Check sheet for the modelled part. Datum: model origin and axes. Units: mm. A direction names the side the tool comes from. Give positions to 0.01 mm unless a question says otherwise; leave off trailing zeros. Order: outer loops, then holes, each group sorted by start corner. A loop starts at its lowest first (then second) coordinate and runs counter-clockwise, first axis right, second up.
from build123d import *

# Parameters (mm, degrees)
F1_DEPTH     = 16.25
F2_DEPTH     = 25
F3_START     = 24
F3_DEPTH     = 1
F4_START     = 17
F4_DEPTH     = 8
F5_T1_DEPTH  = 88.2485217467
F5_T3_DEPTH  = 96.2485217467
F5_T5_DEPTH  = 88.9985217467
F5_T10_DEPTH = 96.5839074706
F5_T15_DEPTH = 88.4985217467
F5_T20_DEPTH = 86.4985217467
F5_T23_ANGLE = 359.64
F5_T25_ANGLE = 359.64


# Not quite as in the source:
# - a fillet or chamfer that OpenCascade refuses, or shapes differently, is made with other operations: its cross-section is extruded or revolved along the edge and cut away or added


with BuildPart() as f1:
    # F0 (on Top) → F1 (new body)
    with BuildSketch(Plane.XY):
        with BuildLine():
            Line((-8.75, -5.75), (-7, -5.75))
            Line((-7, -5.75), (-7, 6.3353857239))
            Line((-7, 6.3353857239), (-9.0223743914, 8.3577601154))
            Line((-9.0223743914, 8.3577601154), (-9.0223743914, 14.1793463062))
            Line((-9.0223743914, 14.1793463062), (-5.6981157623, 15.6555524338))
            Line((-5.6981157623, 15.6555524338), (-1.1670593175, 5.4520969645))
            Line((-1.1670593175, 5.4520969645), (-5, 3.75))
            Line((-5, 3.75), (-5, 1.75))
            ThreePointArc((-5, 1.75), (-3.7625631329, 1.2374368671), (-3.25, 0))
            ThreePointArc((-3.25, 0), (-3.7625631329, -1.2374368671), (-5, -1.75))
            Line((-5, -1.75), (-5, -5.75))
            Line((-5, -5.75), (-2, -5.75))
            Line((-2, -5.75), (-2, -6.25))
            Line((-2, -6.25), (-1, -6.25))
            Line((-1, -6.25), (-1, 10.0037865203))
            Line((-1, 10.0037865203), (-6.1024322628, 21.4939193431))
            Line((-6.1024322628, 21.4939193431), (-12.5, 18.652946438))
            Line((-12.5, 18.652946438), (-12.5, 0.25))
            Line((-12.5, 0.25), (-8.75, 0.25))
            Line((-8.75, 0.25), (-8.75, -5.75))
        make_face()
    extrude(amount=F1_DEPTH)

    # F0 (on Top) → F2 (join)
    with BuildSketch(Plane.XY):
        Polygon((1, 5.5), (-1, 10.0037865203), (-1, -6.25), (1, -6.25), align=None)
    extrude(amount=F2_DEPTH)



with BuildPart() as f2:
    # F0 (on Top) → F2, piece 2 (new body)
    with BuildSketch(Plane.XY):
        with BuildLine():
            Line((6, 5.5), (3, 5.5))
            Line((3, 5.5), (3, 1.75))
            ThreePointArc((3, 1.75), (4.75, 0), (3, -1.75))
            Line((3, -1.75), (3, -6.25))
            Line((3, -6.25), (6, -6.25))
            Line((6, -6.25), (6, 5.5))
        make_face()
    extrude(amount=F2_DEPTH)


with BuildPart() as f1_1:
    add(f1.part)

    add(f2.part)  # F3 merges F2
    # F0 (on Top) → F3 (join)
    with BuildSketch(Plane.XY.offset(F3_START)):
        Polygon((3, 5.5), (1, 5.5), (1, -6.25), (3, -6.25), (3, -1.75), (3, 1.75), align=None)
    extrude(amount=F3_DEPTH)

    # F0 (on Top) → F4 (join)
    with BuildSketch(Plane.XY.offset(F4_START)):
        with BuildLine():
            ThreePointArc((3, -1.75), (4.75, 0), (3, 1.75))
            Line((3, 1.75), (3, -1.75))
        make_face()
    extrude(amount=F4_DEPTH)

    # F5: chamfer of 16.25 x 0.5 on 8 edges, made by hand

    # F5_s2 → F5_t1 (cut)
    with BuildSketch(Plane.XZ.offset(-47.7492608733)):
        Polygon((3.5, 0), (3, 16.25), (3, 0), align=None)
    extrude(amount=F5_T1_DEPTH, mode=Mode.SUBTRACT)

    # F5_s4 → F5_t3 (cut)
    with BuildSketch(Plane.XZ.offset(-47.7492608733)):
        Polygon((0.5, 0), (1, 16.25), (1, 0), align=None)
    extrude(amount=F5_T3_DEPTH, mode=Mode.SUBTRACT)

    # F5_s6 → F5_t5 (cut)
    with BuildSketch(Plane.XZ.offset(-40.4992608733)):
        Polygon((3.5, 0), (3, 16.25), (3, 0), align=None)
    extrude(amount=F5_T5_DEPTH, mode=Mode.SUBTRACT)


with BuildPart() as f5_tool8:
    # F5_s9 → F5_t10 (new body)
    with BuildSketch(Plane.XZ.offset(47.9992608733)):
        Polygon((-7, 16.25), (-7.5, 0), (-7, 0), align=None)
    extrude(amount=-F5_T10_DEPTH)

    split(bisect_by=Plane(origin=(-0.332307138, -0.332307138, 0), x_dir=(0, 0, 1), z_dir=(-0.7071067812, -0.7071067812, 0)), keep=Keep.TOP)


with BuildPart() as f1_2:
    add(f1_1.part)

    # F5_t7: cut F5_tool8
    add(f5_tool8.part, mode=Mode.SUBTRACT)


with BuildPart() as f5_tool13:
    # F5_s14 → F5_t15 (new body)
    with BuildSketch(Plane.XZ.offset(-40.4992608733)):
        Polygon((-5, 16.25), (-4.5, 0), (-5, 0), align=None)
    extrude(amount=F5_T15_DEPTH)

    split(bisect_by=Plane(origin=(1.0474931823, 0.4651611161, 0), x_dir=(0, 0, 1), z_dir=(-0.9139382482, -0.4058532722, 0)), keep=Keep.TOP)


with BuildPart() as f1_3:
    add(f1_2.part)

    # F5_t12: cut F5_tool13
    add(f5_tool13.part, mode=Mode.SUBTRACT)


with BuildPart() as f5_tool18:
    # F5_s19 → F5_t20 (new body)
    with BuildSketch(Plane.XZ.offset(-45.9992608733)):
        Polygon((-5, 16.25), (-4.5, 0), (-5, 0), align=None)
    extrude(amount=F5_T20_DEPTH)

    split(bisect_by=Plane(origin=(1.0474931823, 0.4651611161, 0), x_dir=(0, 0, 1), z_dir=(-0.9139382482, -0.4058532722, 0)), keep=Keep.TOP)


with BuildPart() as f1_4:
    add(f1_3.part)

    # F5_t17: cut F5_tool18
    add(f5_tool18.part, mode=Mode.SUBTRACT)

    # F5_s22 → F5_t23 (revolve, cut)
    with BuildSketch(Plane(origin=(-4.93479e-05, -0.0157078599, 0), x_dir=(0, 0, 1), z_dir=(-0.0031415875, -0.9999950652, 0))):
        Polygon((16.25, 6.749975326), (0, 7.249975326), (0, 6.749975326), align=None)
    revolve(axis=Axis((-5, 0, 0), (0, 0, -1)), revolution_arc=F5_T23_ANGLE, mode=Mode.SUBTRACT)

    # F5_s24 → F5_t25 (revolve, cut)
    with BuildSketch(Plane(origin=(2.96087e-05, 0.0094247159, 0), x_dir=(0, 0, 1), z_dir=(-0.0031415875, -0.9999950652, 0))):
        Polygon((0, -0.7499851956), (16.25, -1.2499851956), (0, -1.2499851956), align=None)
    revolve(axis=Axis((3, 0, 0), (0, 0, -1)), revolution_arc=F5_T25_ANGLE, mode=Mode.SUBTRACT)


solid = f1_4.part
1) Section check D-D, the plane z = 14.5. Record the cut outline in (x, y).
Recorded:
outline: (-12.5, 0.25) - (-8.75, 0.25) - (-8.75, -5.75) - (-7.05, -5.75) - (-7.05, 6.39) - (-9.02, 8.36) - (-9.02, 14.18) - (-5.7, 15.66) - (-1.17, 5.45) - (-4.95, 3.77) - (-4.95, 1.8) arc R1.8 cw to (-4.95, -1.8) - (-4.95, -5.75) - (-2, -5.75) - (-2, -6.25) - (0.95, -6.25) - (0.95, 5.62) - (-6.1, 21.49) - (-12.5, 18.65) - close; (3.05, -6.25) - (6, -6.25) - (6, 5.5) - (3.05, 5.5) - (3.05, 1.8) arc R1.8 cw to (3.05, -1.8) - close
2) Depth check by flat-ended pin: pin 1 Ø4 at (x, z) = (2.5, 16.5) entering from +Y; pin 2 Ø0.9 at (x, z) = (-3.5, 8.5) entering from -Y; pin 3 Ø2.5 at (y, z) = (-1, 22.5) entering from -X. Enter the tip coordinate at first touch or a pass-through.
Recorded:
pin 1: stops at y = 6.63
pin 2: stops at y = -5.75
pin 3: stops at x = -1
3) Set-up check for faces 1 (the face through (-9, 8, 16.25)), 2 (the face through (5, 5.5, 12)), 3 (the face through (-3.06, 4.61, 8.01)), 4 (the face through (-8, -5.75, 8)): record each of +Z, -Z, +X, -X, +Y, -Y from which the full face is reachable in a straight line by a thin tool's end or side.
Recorded:
face 1: +Z, -X, +Y, -Y
face 2: +Z, -Z, +X, +Y
face 3: +Z, -Z
face 4: +Z, -Z, -X, -Y
4) Section check B-B, the plane z = 10.25. Record the cut outline in (x, y), then the cut area to 3 significant figures.
Recorded:
outline: (-12.5, 0.25) - (-8.75, 0.25) - (-8.75, -5.75) - (-7.18, -5.75) - (-7.18, 6.52) - (-9.02, 8.36) - (-9.02, 14.18) - (-5.7, 15.66) - (-1.17, 5.45) - (-4.82, 3.83) - (-4.82, 1.93) arc R1.93 cw to (-4.82, -1.93) - (-4.82, -5.75) - (-2, -5.75) - (-2, -6.25) - (0.82, -6.25) - (0.82, 5.92) - (-6.1, 21.49) - (-12.5, 18.65) - close; (3.18, -6.25) - (6, -6.25) - (6, 5.5) - (3.18, 5.5) - (3.18, 1.93) arc R1.93 cw to (3.18, -1.93) - close
area: 221 mm2
5) Draft check along X on faces 5 (the face through (2, 0, 24)), 6 (the face through (-4, -5.75, 8)), 7 (the face through (6, 0, 12)), 8 (the face through (-9.26, 20.09, 8.01)). Enter one of: +X half, -X half, draft (parallel to the pull), parting line (faces both ways), or undercut.
Recorded:
face 5: undercut
face 6: draft
face 7: +X half
face 8: -X half
6) Material ranges on L1, parallel to X at y = 4.75, z = 22.5; L2, parallel to X at y = 3.75, z = 1; L3, parallel to X at y = 4, z = 2, recorded low to high.
Recorded:
L1: x = -1 to 1, 3 to 6
L2: x = -12.5 to -7.47, -4.53 to 0.53, 3.47 to 6
L3: x = -12.5 to -7.44, -4.44 to 0.56, 3.44 to 6
7) Section check A-A, the plane z = 20.5. Record the cut outline in (x, y).
Recorded:
outline: (-1, -6.25) - (1, -6.25) - (1, 5.5) - (-1, 10) - close; (3, -6.25) - (6, -6.25) - (6, 5.5) - (3, 5.5) - close
8) Section check C-C, the plane x = 2.5. Record the cut outline in (y, z), then the cut area to 4 significant figures.
Recorded:
outline: (-6.25, 24) - (5.5, 24) - (5.5, 25) - (-6.25, 25) - close
area: 11.75 mm2
